Source: CAD feature listing. Evaluate the final solid. Frame: model axes, mm. Give positions to 0.01 mm unless a question says otherwise; leave off trailing zeros. Order: outer loops, then holes, each group sorted by start corner. A loop starts at its lowest first (then second) coordinate and runs counter-clockwise, first axis right, second up. Notation, with made-up numbers: M -12,12 L 16,12 A24 ccw 16,46 Z; hole C 25,-39.75 d1. An arc over 180 degrees is marked long. Return JSON: item names as keys, results as strings.
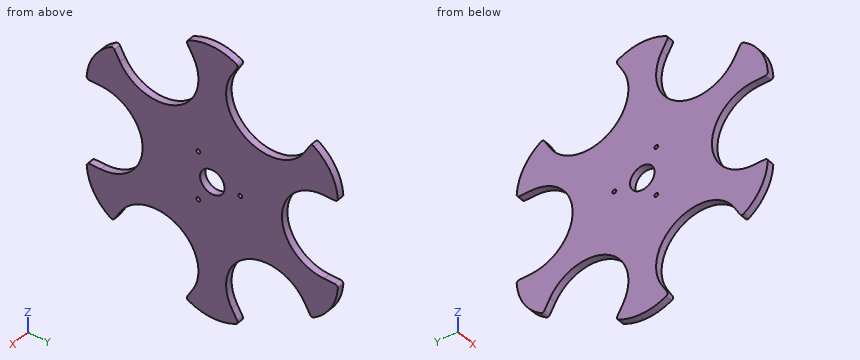
from build123d import *

# Parameters (mm, degrees)
SKETCH1_R                       = 11.110595
BOSS_EXTRUDE1_DEPTH             = 6.35
F_9_64_0_14063_DIAMETER_HOLE1_D = 3.572002
CIRPATTERN1_COUNT               = 3
FILLET1_R                       = 2.54


with BuildPart() as part:
    # Sketch1 → Boss-Extrude1 (new body)
    with BuildSketch(Plane(origin=(0, 0, 0), x_dir=(0, 0, -1), z_dir=(1, 0, 0))):
        with BuildLine():
            Line((68.801578457, 83.832170471), (79.800101085, 90.182170471))
            ThreePointArc((79.800101085, 90.182170471), (62.217829583, 107.764441974), (38.200000054, 114.2))
            Line((38.200000054, 114.2), (38.200000054, 101.5))
            ThreePointArc((38.200000054, 101.5), (0, 63.299999946), (-38.200000054, 101.5))
            Line((-38.200000054, 101.5), (-38.200000054, 114.2))
            ThreePointArc((-38.200000054, 114.2), (-62.217829583, 107.764441974), (-79.800101085, 90.182170471))
            Line((-79.800101085, 90.182170471), (-68.801578457, 83.832170471))
            ThreePointArc((-68.801578457, 83.832170471), (-54.819408013, 31.649999973), (-107.001578511, 17.667829529))
            Line((-107.001578511, 17.667829529), (-118.000101139, 24.017829529))
            ThreePointArc((-118.000101139, 24.017829529), (-124.435659165, 0), (-118.000101139, -24.017829529))
            Line((-118.000101139, -24.017829529), (-107.001578511, -17.667829529))
            ThreePointArc((-107.001578511, -17.667829529), (-54.819408013, -31.649999973), (-68.801578457, -83.832170471))
            Line((-68.801578457, -83.832170471), (-79.800101085, -90.182170471))
            ThreePointArc((-79.800101085, -90.182170471), (-62.217829583, -107.764441974), (-38.200000054, -114.2))
            Line((-38.200000054, -114.2), (-38.200000054, -101.5))
            ThreePointArc((-38.200000054, -101.5), (0, -63.299999946), (38.200000054, -101.5))
            Line((38.200000054, -101.5), (38.200000054, -114.2))
            ThreePointArc((38.200000054, -114.2), (62.217829583, -107.764441974), (79.800101085, -90.182170471))
            Line((79.800101085, -90.182170471), (68.801578457, -83.832170471))
            ThreePointArc((68.801578457, -83.832170471), (54.819408013, -31.649999973), (107.001578511, -17.667829529))
            Line((107.001578511, -17.667829529), (118.000101139, -24.017829529))
            ThreePointArc((118.000101139, -24.017829529), (124.435659165, 0), (118.000101139, 24.017829529))
            Line((118.000101139, 24.017829529), (107.001578511, 17.667829529))
            ThreePointArc((107.001578511, 17.667829529), (54.819408013, 31.649999973), (68.801578457, 83.832170471))
        make_face()
        Circle(SKETCH1_R, mode=Mode.SUBTRACT)
    extrude(amount=BOSS_EXTRUDE1_DEPTH)

    # 9/64 (0.14063) Diameter Hole1 (through all)
    with Locations(Plane(origin=(6.35, 0, 0), x_dir=(0, 0, -1), z_dir=(1, 0, 0))):
        with Locations((0, 25.4)):
            f_9_64_0_14063_diameter_hole1 = Hole(F_9_64_0_14063_DIAMETER_HOLE1_D / 2)

    # CirPattern1: 9/64 (0.14063) Diameter Hole1 ×3 about axis
    cirpattern1_axis = Axis((0, 0, 0), (1, 0, 0))
    for i in range(1, CIRPATTERN1_COUNT):
        add(f_9_64_0_14063_diameter_hole1.rotate(cirpattern1_axis, i * 360 / CIRPATTERN1_COUNT), mode=Mode.SUBTRACT)

    # Fillet1
    fillet1_edges = [part.edges().sort_by_distance(p)[0] for p in [
        (3.175, 114.2, -38.200000054),
        (3.175, 90.182170471, -79.800101085),
        (3.175, 24.017829529, -118.000101139),
        (3.175, -24.017829529, -118.000101139),
        (3.175, -90.182170471, -79.800101085),
        (3.175, -114.2, -38.200000054),
        (3.175, -114.2, 38.200000054),
        (3.175, -90.182170471, 79.800101085),
        (3.175, -24.017829529, 118.000101139),
        (3.175, 24.017829529, 118.000101139),
        (3.175, 90.182170471, 79.800101085),
        (3.175, 114.2, 38.200000054),
    ]]
    fillet(fillet1_edges, radius=FILLET1_R)


solid = part.part
1. Ray query, probe 1 along Y at (x, z) = (4, 0); probe 2 along Y at (x, z) = (4.5, 58); probe 3 along Z at (x, y) = (1.25, -20.5). Return the intervals inside material, ascending.
Evaluation:
{"probe 1": "y = -63.3 to -11.11, 11.11 to 23.61, 27.19 to 63.3", "probe 2": "y = -109.93 to -74.52, -26.98 to 26.98, 74.52 to 109.93", "probe 3": "z = -119.84 to -111.91, -64.57 to 64.57, 111.91 to 119.84"}
2. Section query D-D (x = 1.5). State how many separate pieces and enclosed holes the cut face has, then the cut area to 3 significant figures.
Evaluation:
{"separate pieces": "1", "enclosed holes": "4", "area": "24,400 mm^2"}
3. Section query A-A (y = 0). Return loops of the section in (x, z).
Evaluation:
{"outline": "M 0,-124.44 L 6.35,-124.44 L 6.35,-11.11 L 0,-11.11 Z; M 0,11.11 L 6.35,11.11 L 6.35,124.44 L 0,124.44 Z"}
4. Section query B-B (z = 60.5). Return loops of the section in (x, y).
Evaluation:
{"outline": "M 0,-108.71 L 6.35,-108.71 L 6.35,-77.37 L 0,-77.37 Z; M 0,-24.13 L 6.35,-24.13 L 6.35,24.13 L 0,24.13 Z; M 0,77.37 L 6.35,77.37 L 6.35,108.71 L 0,108.71 Z"}
5. Section query C-C (y = -97). Return loops of the section in (x, z), then the cut area to 3 significant figures.
Evaluation:
{"outline": "M 0,-75.03 L 6.35,-75.03 L 6.35,-37.93 L 0,-37.93 Z; M 0,37.93 L 6.35,37.93 L 6.35,75.03 L 0,75.03 Z", "area": "471 mm^2"}
